For this review, take the finished solid that the model builds, in its own axes (mm). Face numbers are marked on the shaded views. Give positions to 0.01 mm unless a question says otherwise; leave off trailing zeros. Write each loop counter-clockwise with the first axis right and the second up, starting at its lowest first coordinate (ties: lowest second). Pieces come first, ordered by that corner, then holes. Notation, with made-up numbers: (35.25, 3) -> (52.25, 3) arc R25 cw to (52.25, 23) -> close; hole circle Ø4 at (-13.5, 43.5). An arc over 180 degrees is marked (long way). Return JSON: item names as keys, results as strings.
from build123d import *

# Parameters (mm, degrees)
SKETCH1_W           = 110
SKETCH1_H           = 180
BOSS_EXTRUDE1_DEPTH = 1.25
BOSS_EXTRUDE3_DEPTH = 2.5


with BuildPart() as part:
    # Sketch1 → Boss-Extrude1 (new, symmetric)
    with BuildSketch(Plane(origin=(0, 0, 0), x_dir=(1, 0, 0), z_dir=(0, 1, 0))):
        Rectangle(SKETCH1_W, SKETCH1_H)
    extrude(amount=BOSS_EXTRUDE1_DEPTH, both=True)

    # Sketch2 → Boss-Extrude3 (add)
    with BuildSketch(Plane(origin=(0, 1.25, 0), x_dir=(1, 0, 0), z_dir=(0, 1, 0))):
        Polygon((53.5, -88.5), (-53.5, -88.5), (-53.5, -71.5), (-51.6, -71.5), (-51.6, -86.5), (51.6, -86.5), (51.6, -73), (53.5, -73), align=None)
        Polygon((53.5, 88.5), (-53.5, 88.5), (-53.5, -29.5), (-51.6, -29.5), (-51.6, 86.5), (51.6, 86.5), (51.6, -19), (53.5, -19), align=None)
    extrude(amount=BOSS_EXTRUDE3_DEPTH)


solid = part.part
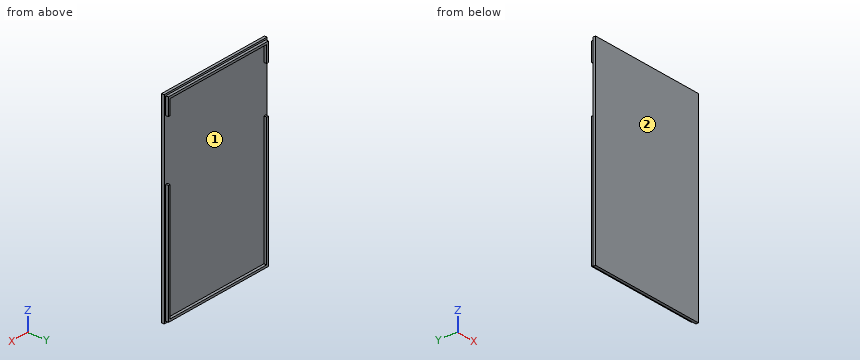
1. For pin 1 (0.8 mm diameter, centred on y = 3, z = -43.5, fed in from -X); pin 2 (2 mm diameter, centred on y = 3, z = 80, fed in from +X); pin 3 (0.6 mm diameter, centred on x = -52.5, y = 3, fed in from +Z), all flat-tipped, find the tip position at first contact; note any pin that passes through.
Results found:
{"pin 1": "stops at x = -53.5", "pin 2": "stops at x = 53.5", "pin 3": "stops at z = 88.5"}
2. Add section B-B, the plane z = -17. State the section outline as (x, y) points, plus the area to 4 significant figures.
Results found:
{"outline": "(-55, -1.25) -> (55, -1.25) -> (55, 1.25) -> (53.5, 1.25) -> (53.5, 3.75) -> (51.6, 3.75) -> (51.6, 1.25) -> (-51.6, 1.25) -> (-51.6, 3.75) -> (-53.5, 3.75) -> (-53.5, 1.25) -> (-55, 1.25) -> close", "area": "284.5 mm²"}
3. The part is to be moulded in two halves that separate along X. For the marked faces 1 and 2, say which applies: +X half, -X half, draft (parallel to the pull), parting line (faces both ways), or undercut.
Results found:
{"face 1": "undercut", "face 2": "draft"}
4. Add section A-A, the plane y = 2. State the section outline as (x, z) points.
Results found:
{"outline": "(-53.5, -88.5) -> (53.5, -88.5) -> (53.5, 19) -> (51.6, 19) -> (51.6, -86.5) -> (-51.6, -86.5) -> (-51.6, 29.5) -> (-53.5, 29.5) -> close; (-53.5, 71.5) -> (-51.6, 71.5) -> (-51.6, 86.5) -> (51.6, 86.5) -> (51.6, 73) -> (53.5, 73) -> (53.5, 88.5) -> (-53.5, 88.5) -> close"}
5. Add section D-D, the plane z = 61.5. State the section outline as (x, y) points, plus the area to 3 significant figures.
Results found:
{"outline": "(-55, -1.25) -> (55, -1.25) -> (55, 1.25) -> (-55, 1.25) -> close", "area": "275 mm²"}
6. Add section C-C, the plane x = -40. State the section outline as (y, z) points, plus the area to 3 significant figures.
Results found:
{"outline": "(-1.25, -90) -> (1.25, -90) -> (1.25, -88.5) -> (3.75, -88.5) -> (3.75, -86.5) -> (1.25, -86.5) -> (1.25, 86.5) -> (3.75, 86.5) -> (3.75, 88.5) -> (1.25, 88.5) -> (1.25, 90) -> (-1.25, 90) -> close", "area": "460 mm²"}
7. To check wall thickness, follow probe 1 along Z at (x, y) = (18, 2.4); probe 2 along X at (y, z) = (2.65, 75.5); probe 3 along Y at (x, z) = (-46.5, -18). State the ranges of each line that lie inside material, in increasing order.
Results found:
{"probe 1": "z = -88.5 to -86.5, 86.5 to 88.5", "probe 2": "x = -53.5 to -51.6, 51.6 to 53.5", "probe 3": "y = -1.25 to 1.25"}
